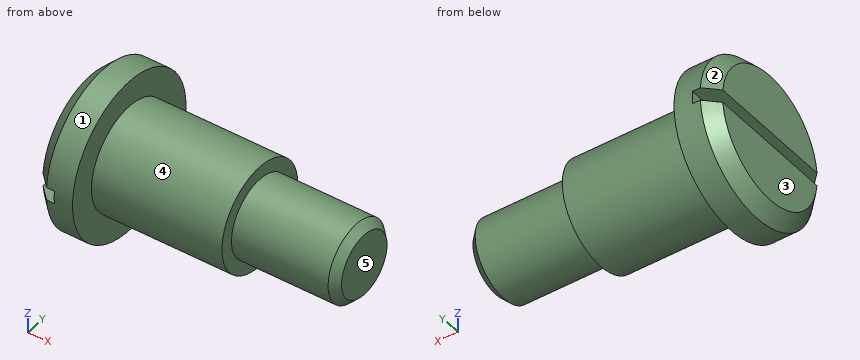
Autodesk Inventor part; units mm, degrees
ref_plane "YZ Plane" through (0, 0, 0) normal (1, 0, 0) x (0, 1, 0)
ref_plane "XZ Plane" through (0, 0, 0) normal (0, 1, 0) x (-1, 0, 0)
ref_plane "XY Plane" through (0, 0, 0) normal (0, 0, 1) x (1, 0, 0)
sketch "Skizze1" plane through (0, 0, 0) normal (0, 0, 1) x (1, 0, 0)
  line L0 (-2.1, 0) -> (12.6, 0)
  line L1 (0, -0.6) -> (0, 3.6)
  line L2 (0, 0) -> (0, 3)
  line L3 (0, 3) -> (1.5, 3)
  line L4 (1.5, 3) -> (1.5, 2)
  line L5 (1.5, 2) -> (6.5, 2)
  line L6 (6.5, 2) -> (6.5, 1.5)
  line L7 (6.5, 1.5) -> (10.5, 1.5)
  line L8 (10.5, 1.5) -> (10.5, 0)
  line L9 (10.5, 0) -> (0, 0)
  dimension "d0" = 6
  dimension "d1" = 4
  dimension "d2" = 3
  dimension "d3" = 10.5
  dimension "d4" = 4
  dimension "d5" = 9
revolve "Umdrehung1" add sketch "Skizze1" angle 360 about axis through (-10, 0, 0) along (1, 0, 0)
thread "Gewinde1"
chamfer "Fase1" distance 0.3 angle 45 1 edges at (10.5, -1.5, 0)
chamfer "Fase2" distance 0.5 angle 45 1 edges at (0, -3, 0)
sketch "Skizze2" plane through (0, 0, 0) normal (-1, 0, 0) x (0, 0, 1)
  line L0 (0, -4.2) -> (0, 4.2)
  line L1 (-4.2, 0) -> (4.2, 0)
  circle A0 centre (0, 0) radius 3
  circle A1 centre (0, 0) radius 3
  line L2 (-0.25, 2.9896) -> (-0.25, -2.9896)
  line L3 (0.25, -2.9896) -> (0.25, 2.9896)
  arc A2 (-0.25, -2.9896) -> (0.25, -2.9896) centre (0, 0) ccw
  arc A3 (0.25, 2.9896) -> (-0.25, 2.9896) centre (0, 0) ccw
  dimension "d15" = 0.5
extrude "Extrusion1" cut sketch "Skizze2" against normal blind 0.8 contours A0 L2 L1 L0 | L0 L1 L3 A0 | L1 L2 A0 L0 | L0 A0 L3 L1
properties part number "Zapfen"
For this review, take the finished solid that the model builds, in its own axes (mm). Face numbers are marked on the shaded views. A direction names the side the tool comes from. Coordinates: 2 decimals unless noted, no trailing zeros. Order: outer loops, then holes, each group sorted by start corner. A loop starts at its lowest first (then second) coordinate and runs counter-clockwise, first axis right, second up. Notation, with made-up numbers: (72.5, 15.25) - (100.5, 15.25) arc R12 ccw to (100.5, 33.25) - close; hole circle Ø1 at (78.5, -2). An arc over 180 degrees is marked (long way). Answer as a JSON object with one key per item and string values. Group by question number.
1. We need section B-B on z = 0. State the section outline as (x, y) points, then the cut area to 3 significant figures.
2. We need section A-A on y = 0. State the section outline as (x, z) points, then the cut area to 3 significant figures.
3. The part is to be moulded in two halves that separate along Z. For the marked faces 1, 2 and 3, say which applies: pulls with the +Z half, pulls with the -Z half, needs draft (parallel to the pull), parting line crosses it, or undercut.
4. For probe 1 along X at (y, z) = (-2.7, -0.2); probe 2 along X at (y, z) = (-0.95, -1.6); probe 3 along Z at (x, y) = (0.75, 2.75), list the stretches that pass through material, from the lowest coordinate up.
5. We need section D-D on x = 3. State the section outline as (y, z) points.
6. We need section C-C on x = 9. State the section outline as (y, z) points, then the cut area to 3 significant figures.
7. For the marked faces 4 and 5, list the 3-axis set-ups (+Z, -Z, +X, -X, +Y, -Y) from which the entire face can be reached by the end or side of a thin tool; tool diameter is ignored.
8. Clearance check with a flat-ended pin moving along its axis: P1, Ø2, axis at y = -1, z = -2.5, coming from the +X side. State where the tip first meets the part, or that it passes through.
Final values:
{
 "1": {"outline": "(0.8, -3) - (1.5, -3) - (1.5, -2) - (6.5, -2) - (6.5, -1.5) - (10.2, -1.5) - (10.5, -1.2) - (10.5, 1.2) - (10.2, 1.5) - (6.5, 1.5) - (6.5, 2) - (1.5, 2) - (1.5, 3) - (0.8, 3) - close", "area": "36.1 mm²"},
 "2": {"outline": "(0, -2.5) - (0.5, -3) - (1.5, -3) - (1.5, -2) - (6.5, -2) - (6.5, -1.5) - (10.2, -1.5) - (10.5, -1.2) - (10.5, 1.2) - (10.2, 1.5) - (6.5, 1.5) - (6.5, 2) - (1.5, 2) - (1.5, 3) - (0.5, 3) - (0, 2.5) - (0, 0.25) - (0.8, 0.25) - (0.8, -0.25) - (0, -0.25) - close", "area": "40.3 mm²"},
 "3": {"face 1": "parting line crosses it", "face 2": "pulls with the +Z half", "face 3": "needs draft"},
 "4": {"probe 1": "0.8 to 1.5", "probe 2": "0 to 6.5", "probe 3": "-1.2 to -0.25, 0.25 to 1.2"},
 "5": {"outline": "circle Ø4 at (0, 0)"},
 "6": {"outline": "circle Ø3 at (0, 0)", "area": "7.07 mm²"},
 "7": {"face 4": "+X", "face 5": "+Z, -Z, +X, +Y, -Y"},
 "8": {"P1": "x = 6.5"}
}
